from build123d import *

# Parameters (mm, degrees)
BOSS_EXTRUDE1_DEPTH = 8
SKETCH4_R           = 6
BOSS_EXTRUDE2_DEPTH = 104


with BuildPart() as part:
    # Sketch2 → Boss-Extrude1 (new body)
    with BuildSketch(Plane.XY):
        Polygon((-17.678131714, 1.510354203), (0, 17.742533943), (16.23217974, 0.064402229), (-1.445951974, -16.167777511), align=None)
    extrude(amount=-BOSS_EXTRUDE1_DEPTH)

    # Sketch4 → Boss-Extrude2 (add)
    with BuildSketch(Plane.XY):
        Circle(SKETCH4_R)
    extrude(amount=-BOSS_EXTRUDE2_DEPTH)


solid = part.part
Design review of the part built by this model. Coordinates are the model's own, in mm. A direction names the side the tool comes from. Round coordinates to 2 decimals unless told otherwise and drop trailing zeros. Write each loop counter-clockwise with the first axis right and the second up, starting at its lowest first coordinate (ties: lowest second). Pieces come first, ordered by that corner, then holes. Notation, with made-up numbers: M 35.5,16 L 44.5,16 A20 ccw 44.5,34 Z; hole C 4,64.5 d9. An arc over 180 degrees is marked long. One line per item, written item: value. Start each with the question number.
1. Clearance check with flat-ended pins moving along their axes: P1, Ø17, axis at x = -7, y = 3, coming from the -Z side; P2, Ø4, axis at y = 0.5, z = -84.5, coming from the +X side; P3, Ø1.5, axis at x = -1, y = 10.5, coming from the -Z side. State where each tip first meets the part, or that it passes through.
2. Take a section at A-A on z = -7. State the section outline as (x, y) points.
3. Take a section at B-B on x = -4. State the section outline as (y, z) points, then the cut area to 3 significant figures.
4. For faces 1 (the face through (7.517, -7.938, -3.944)), 2 (the face through (-6, 0, -55)), list the 3-axis set-ups (+Z, -Z, +X, -X, +Y, -Y) from which the entire face can be reached by the end or side of a thin tool; tool diameter is ignored.
5. To check wall thickness, follow probe 1 along Z at (x, y) = (-7, -5.5); probe 2 along Y at (x, z) = (8, -4.5); probe 3 along Y at (x, z) = (-2, -39). State the ranges of each line that lie inside material, in increasing order. Write a range as from..to.
6. Take a section at D-D on z = -71. State the section outline as (x, y) points.
7. Take a section at C-C on y = -2. State the section outline as (x, z) points, then the cut area to 3 significant figures.
Computed:
1. P1: stops at z = -104
1. P2: stops at x = 6
1. P3: stops at z = -8
2. outline: M -17.68,1.51 L -1.45,-16.17 L 16.23,0.06 L 0,17.74 Z
3. outline: M -13.39,-8 L -4.47,-8 L -4.47,-104 L 4.47,-104 L 4.47,-8 L 14.07,-8 L 14.07,0 L -13.39,0 Z
3. area: 1,080 mm²
4. face 1: +Z, -Z, +X, -Y
4. face 2: -Z
5. probe 1: z = -8..0
5. probe 2: y = -7.49..9.03
5. probe 3: y = -5.66..5.66
6. outline: C 0,0 d12
7. outline: M -14.45,-8 L -5.66,-8 L -5.66,-104 L 5.66,-104 L 5.66,-8 L 13.98,-8 L 13.98,0 L -14.45,0 Z
7. area: 1,310 mm²
